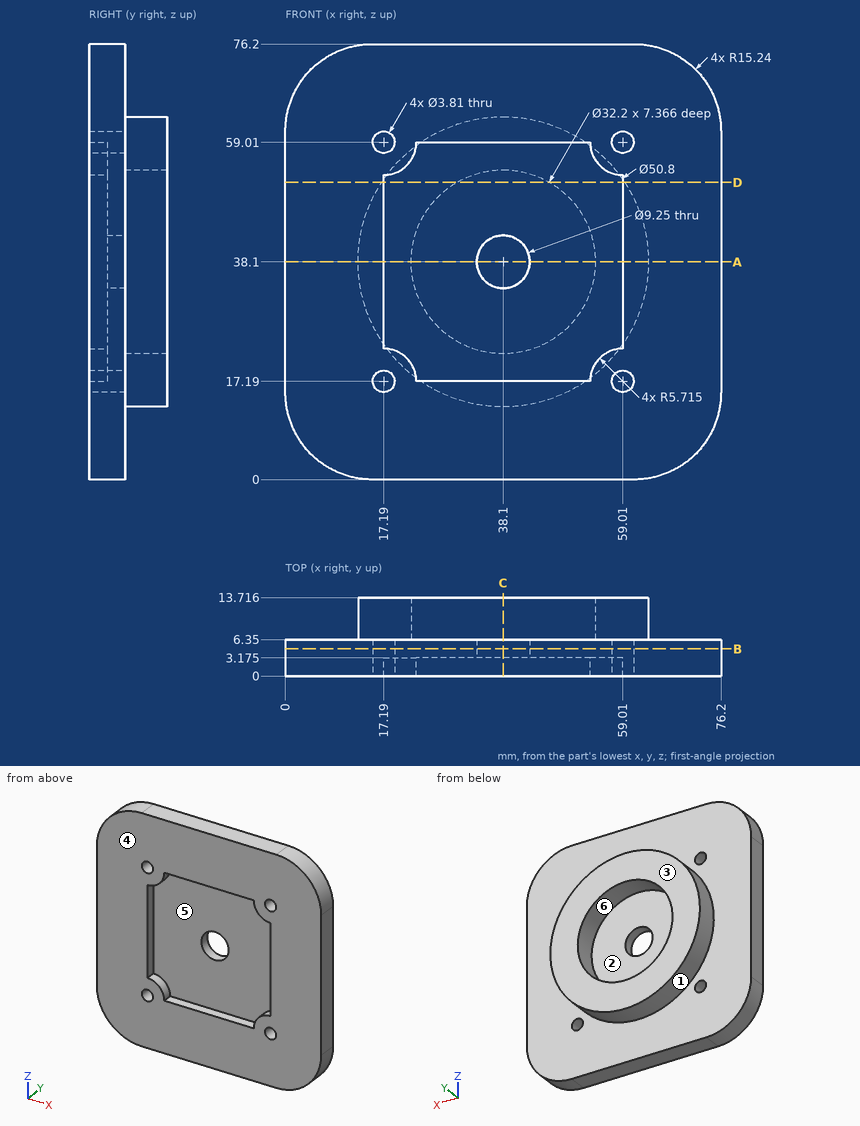
Design review of the part shown in the three views and the two pictorial views. Dimensions are in mm from the part's minimum x, y and z. A direction names the side the tool comes from. Give positions to 0.01 mm unless a question says otherwise; leave off trailing zeros. Write each loop counter-clockwise with the first axis right and the second up, starting at its lowest first coordinate (ties: lowest second). Pieces come first, ordered by that corner, then holes. Notation, with made-up numbers: (52.25, -35) -> (59.25, -35) arc R9 cw to (59.25, -28) -> close; hole circle Ø7 at (58.25, 68.25). An arc over 180 degrees is marked (long way). Answer in a Markdown table with one row per item.
1) Add section C-C on x = 38.1. State the section outline as (y, z) points (3 decimals), plus the area to 3 significant figures.
Worked answers:
| item | result |
|---|---|
| outline | (0, 0) -> (6.35, 0) -> (6.35, 12.7) -> (13.716, 12.7) -> (13.716, 22) -> (6.35, 22) -> (6.35, 33.475) -> (3.175, 33.475) -> (3.175, 17.19) -> (0, 17.19) -> close; (0, 59.01) -> (3.175, 59.01) -> (3.175, 42.725) -> (6.35, 42.725) -> (6.35, 54.2) -> (13.716, 54.2) -> (13.716, 63.5) -> (6.35, 63.5) -> (6.35, 76.2) -> (0, 76.2) -> close |
| area | 459 mm² |
2) For L1, parallel to X at y = 2.5, z = 39.5; L2, parallel to Z at x = 18.5, y = 5, list the stretches that pass through material, from the lowest coordinate up. Write a range as [from, to].
Worked answers:
| item | result |
|---|---|
| L1 | [0, 17.19], [59.01, 76.2] |
| L2 | [0, 15.81], [18.57, 57.63], [60.39, 76.2] |
3) Add section A-A on z = 38.1. State the section outline as (x, y) points (3 decimals).
Worked answers:
| item | result |
|---|---|
| outline | (0, 0) -> (17.19, 0) -> (17.19, 3.175) -> (33.475, 3.175) -> (33.475, 6.35) -> (22, 6.35) -> (22, 13.716) -> (12.7, 13.716) -> (12.7, 6.35) -> (0, 6.35) -> close; (42.725, 3.175) -> (59.01, 3.175) -> (59.01, 0) -> (76.2, 0) -> (76.2, 6.35) -> (63.5, 6.35) -> (63.5, 13.716) -> (54.2, 13.716) -> (54.2, 6.35) -> (42.725, 6.35) -> close |
4) Mouldability with a two-part tool opening along X and no side actions: class the marked faces 1, 2 and 3 as +X half, -X half, draft (parallel to the pull), parting line (faces both ways), or undercut.
Worked answers:
| item | result |
|---|---|
| face 1 | parting line |
| face 2 | undercut |
| face 3 | draft |
5) Add section D-D on z = 52. State the section outline as (x, y) points (3 decimals).
Worked answers:
| item | result |
|---|---|
| outline | (0, 0) -> (17.19, 0) -> (17.19, 3.175) -> (59.01, 3.175) -> (59.01, 0) -> (76.2, 0) -> (76.2, 6.35) -> (59.359, 6.35) -> (59.359, 13.716) -> (46.224, 13.716) -> (46.224, 6.35) -> (29.976, 6.35) -> (29.976, 13.716) -> (16.841, 13.716) -> (16.841, 6.35) -> (0, 6.35) -> close |
6) Add section B-B on y = 4.75. State the section outline as (x, z) points (3 decimals), plus the area to 3 significant figures.
Worked answers:
| item | result |
|---|---|
| outline | (0, 15.24) arc R15.24 ccw to (15.24, 0) -> (60.96, 0) arc R15.24 ccw to (76.2, 15.24) -> (76.2, 60.96) arc R15.24 ccw to (60.96, 76.2) -> (15.24, 76.2) arc R15.24 ccw to (0, 60.96) -> close; hole circle Ø3.81 at (17.19, 17.19); hole circle Ø3.81 at (17.19, 59.01); hole circle Ø9.25 at (38.1, 38.1); hole circle Ø3.81 at (59.01, 17.19); hole circle Ø3.81 at (59.01, 59.01) |
| area | 5,490 mm² |
7) Clearance check with flat-ended pins moving along their axes: P1, Ø3, axis at x = 47, z = 38.5, coming from the +Y side; P2, Ø3.5, axis at x = 17.19, z = 59.01, coming from the -Y side; P3, Ø5, axis at x = 68.5, y = 1.5, coming from the +Z side; P4, Ø12.5, axis at x = 36.5, z = 38, coming from the -Y side (3 decimals). State where each tip first meets the part, or that it passes through.
Worked answers:
| item | result |
|---|---|
| P1 | y = 6.35 |
| P2 | through |
| P3 | z = 75.34 |
| P4 | y = 3.175 |
8) Tool access review of the marked faces 4, 5 and 6: name each direction out of +Z, -Z, +X, -X, +Y, -Y from which nothing blocks a thin tool from reaching the whole face with its end or side.
Worked answers:
| item | result |
|---|---|
| face 4 | +Z, -Z, +X, -X, -Y |
| face 5 | -Y |
| face 6 | +Y |
